Part model, mm, in its own coordinate system. Face numbers are marked on the shaded views. A direction names the side the tool comes from. Coordinates: 2 decimals unless noted, no trailing zeros. Write each loop counter-clockwise with the first axis right and the second up, starting at its lowest first coordinate (ties: lowest second). Pieces come first, ordered by that corner, then holes. Notation, with made-up numbers: M 88.5,84.25 L 139.5,84.25 A24 ccw 139.5,95.25 Z; hole C 57.25,13 d4. An arc over 180 degrees is marked long. Use a Markdown table: item, result. Add a question column.
Q1. Slice it at B-B on z = -24. Write the cut outline in (x, y).
Q2. Wall check: L1, parallel to Y at x = 26, z = 2.5; L2, parallel to Z at x = -24.5, y = 35.5; L3, parallel to Y at x = -27, z = -42. Give the ranges that are in metal, low to high. Write a range as from..to.
Q3. Slice it at A-A on y = 1. Write the cut outline in (x, z), then the cut area to 3 significant figures.
Q4. Slice it at D-D on y = 26. Write the cut outline in (x, z), then the cut area to 3 significant figures.
Q5. Pin check, flat tips, straight feed: pin 1 Ø10 at (x, z) = (-25, -36) entering from -Y; pin 2 Ø24 at (y, z) = (13, 8) entering from -X; pin 3 Ø5 at (y, z) = (-2, -37.5) entering from +X. Stop position of each tip, or through.
Q6. Tool access for the marked faces 5, 6 and 7: list every direction of +Z, -Z, +X, -X, +Y, -Y with a clear straight run to the whole face (end or side of a thin tool).
Q7. Mould opens along Z. For the marked faces 1, 2, 3 and 4 say: released by +Z, released by -Z, zero draft, split by the parting line, or undercut.
Q8. Slice it at C-C on x = -25. Write the cut outline in (y, z).
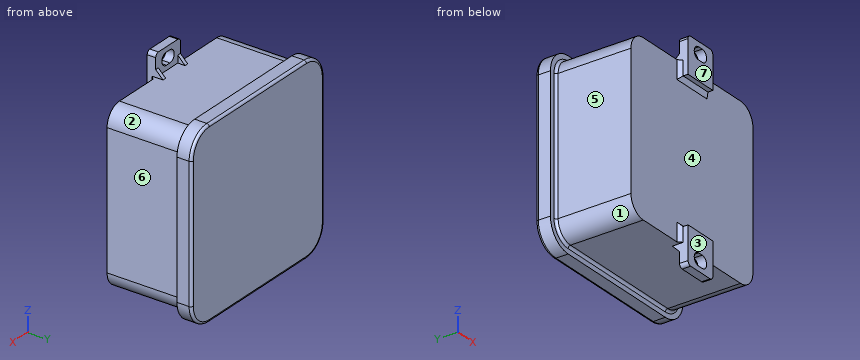
Autodesk Inventor part; units mm, degrees
ref_plane "Work Plane1" through (-1.9723, -3.5, 38.1266) normal (1, 0, 0) x (0, 0, -1)
ref_plane "Work Plane2" through (-29.4723, 30, -5.3734) normal (0, 0, 1) x (1, 0, 0)
ref_plane "YZ Plane" through (0, 0, 0) normal (1, 0, 0) x (0, 1, 0)
sketch "Sketch1" plane through (0, 0, 0) normal (0, 1, 0) x (-1, 0, 0)
  line L0 (36.4723, -39.8734) -> (-32.5277, -39.8734)
  line L1 (-32.5277, -39.8734) -> (-32.5277, 29.1266)
  line L2 (-32.5277, 29.1266) -> (36.4723, 29.1266)
  line L3 (36.4723, 29.1266) -> (36.4723, -39.8734)
  line L4 (36.4723, -39.8734) -> (-32.5277, 29.1266) construction
  line L5 (-32.5277, -39.8734) -> (36.4723, 29.1266) construction
  point P0 (0, 0)
  point P1 (1.9723, -5.3734)
  dimension "d0" = 69
  dimension "d1" = 69
extrude "Extrusion1" add sketch "Sketch1" along normal blind 31
fillet "Fillet1" radius 7 4 edges at (32.5277, 15.5, 29.1266) (-36.4723, 15.5, 29.1266) (-36.4723, 15.5, -39.8734) (32.5277, 15.5, -39.8734)
sketch "Sketch2" plane through (0, 31, 0) normal (0, 1, 0) x (1, 0, 0)
  arc A0 (32.5277, 32.8734) -> (25.5277, 39.8734) centre (25.5277, 32.8734) ccw
  line L0 (25.5277, 39.8734) -> (-29.4723, 39.8734)
  arc A1 (-29.4723, 39.8734) -> (-36.4723, 32.8734) centre (-29.4723, 32.8734) ccw
  line L1 (-36.4723, 32.8734) -> (-36.4723, -22.1266)
  arc A2 (-36.4723, -22.1266) -> (-29.4723, -29.1266) centre (-29.4723, -22.1266) ccw
  line L2 (-29.4723, -29.1266) -> (25.5277, -29.1266)
  arc A3 (25.5277, -29.1266) -> (32.5277, -22.1266) centre (25.5277, -22.1266) ccw
  line L3 (32.5277, -22.1266) -> (32.5277, 32.8734)
  line L4 (-29.4723, 42.8734) -> (25.5277, 42.8734)
  arc A4 (35.5277, 32.8734) -> (25.5277, 42.8734) centre (25.5277, 32.8734) ccw
  line L5 (35.5277, 32.8734) -> (35.5277, -22.1266)
  arc A5 (25.5277, -32.1266) -> (35.5277, -22.1266) centre (25.5277, -22.1266) ccw
  line L6 (25.5277, -32.1266) -> (-29.4723, -32.1266)
  arc A6 (-39.4723, -22.1266) -> (-29.4723, -32.1266) centre (-29.4723, -22.1266) ccw
  line L7 (-39.4723, -22.1266) -> (-39.4723, 32.8734)
  arc A7 (-29.4723, 42.8734) -> (-39.4723, 32.8734) centre (-29.4723, 32.8734) ccw
  point P0 (0, 0)
  dimension "d5" = 3
extrude "Extrusion2" add sketch "Sketch2" along normal blind 6 contours L3 A3 L2 A2 L1 A1 L0 A0 | L4 A4 L5 A5 L6 A6 L7 A7
fillet "Fillet2" radius 1 8 edges at (-1.9723, 31, 29.1266) (-34.422, 31, 27.0763) (-36.4723, 31, -5.3734) (-34.422, 31, -37.8232) (-1.9723, 31, -39.8734) (30.4775, 31, -37.8232) (32.5277, 31, -5.3734) (30.4775, 31, 27.0763)
fillet "Fillet3" radius 1 8 edges at (32.5988, 37, 29.1977) (35.5277, 37, -5.3734) (32.5988, 37, -39.9445) (-1.9723, 37, -42.8734) (-36.5433, 37, -39.9445) (-39.4723, 37, -5.3734) (-36.5433, 37, 29.1977) (-1.9723, 37, 32.1266)
sketch "Sketch3" plane through (0, 0, 0) normal (0, -1, 0) x (1, 0, 0)
  line L0 (32.5277, -32.8734) -> (32.5277, 22.1266)
  line L1 (25.5277, 29.1266) -> (-29.4723, 29.1266)
  line L2 (-36.4723, 22.1266) -> (-36.4723, -32.8734)
  line L3 (-8.9723, 38.1266) -> (5.0277, 38.1266)
  line L4 (5.0277, 38.1266) -> (5.0277, 23.1266)
  line L5 (5.0277, 23.1266) -> (-8.9723, 23.1266)
  line L6 (-8.9723, 23.1266) -> (-8.9723, 38.1266)
  line L7 (-8.9723, 23.1266) -> (-36.4723, 23.1266)
  line L8 (5.0277, 23.1266) -> (32.5277, 23.1266)
  point P0 (0, 0)
  dimension "d10" = 14
  dimension "d12" = 15
  dimension "d13" = 9
extrude "Extrusion3" add sketch "Sketch3" along normal blind 3.5
chamfer "Chamfer1" distance 1.5 angle 45 3 edges at (-8.9723, 0, 26.1266) (-1.9723, 0, 23.1266) (5.0277, 0, 26.1266)
sketch "Sketch4" plane through (0, 0, 0) normal (0, 1, 0) x (1, 0, 0)
  line L0 (5.0277, -29.1266) -> (-8.9723, -29.1266)
  line L1 (-8.9723, -38.1266) -> (5.0277, -38.1266)
  line L2 (-1.9723, -38.1266) -> (-1.9723, -29.1266)
  line L3 (-1.9723, -33.6266) -> (-0.9723, -33.6266)
  line L4 (-1.9723, -33.6266) -> (-2.9723, -33.6266)
  circle A0 centre (-2.9723, -33.6266) radius 2.5
  circle A1 centre (-0.9723, -33.6266) radius 2.5
  line L5 (-2.9723, -31.1266) -> (-0.9723, -31.1266)
  line L6 (-0.9723, -31.1266) -> (-0.9723, -36.1266)
  line L7 (-0.9723, -36.1266) -> (-2.9723, -36.1266)
  line L8 (-2.9723, -36.1266) -> (-2.9723, -31.1266)
  point P0 (0, 0)
  dimension "d21" = 5
  dimension "d22" = 5
  dimension "d19" = 1
  dimension "d20" = 1
extrude "Extrusion4" cut sketch "Sketch4" against normal blind 3.5
sketch "Sketch5" plane through (5.0277, 0, 38.1266) normal (1, 0, 0) x (0, 0, -1)
  line L0 (0, 0) -> (9, 0)
  line L1 (9, 0) -> (9, 30)
  line L2 (9, -1.5) -> (9, 0)
  line L3 (9, 0) -> (9, -1.5)
  line L4 (9, -1.5) -> (9, 0)
  line L5 (9, -1.5) -> (9, 0)
  line L6 (9, 30) -> (9, 0)
  line L7 (6, 0) -> (9, 3)
  line L8 (6, 0) -> (10.2426, 0) construction
  line L9 (6, 0) -> (9, 0)
  line L10 (9, 3) -> (9, 0)
  point P0 (38.1266, 0)
  dimension "d25" = 45
  dimension "d26" = 3
extrude "Extrusion5" add sketch "Sketch5" against normal blind 1.5
ref_plane "Work Plane1" through (-1.9723, -3.5, 38.1266) normal (1, 0, 0) x (0, 0, -1)
mirror "Mirror1" about plane through (-1.9723, -3.5, 38.1266) normal (1, 0, 0) of "Extrusion5"
fillet "Fillet4" radius 1.5 2 edges at (-8.9723, -1.75, 38.1266) (5.0277, -1.75, 38.1266)
ref_plane "Work Plane2" through (-29.4723, 30, -5.3734) normal (0, 0, 1) x (1, 0, 0)
mirror "Mirror2" about plane through (-29.4723, 30, -5.3734) normal (0, 0, 1) of "Extrusion3", "Chamfer1", "Extrusion4", "Extrusion5", "Mirror1", "Fillet4"
ref_plane "Work Plane3" through (-1.9723, -3.5, -48.8734) normal (-1, 0, 0) x (0, 0, 1)
properties part number "power_conduit_box"
Recorded:
| question | item | result |
|---|---|---|
| 1 | outline | M -39.47,31 L -37.47,31 A1 cw -36.47,30 L -36.47,0 L 32.53,0 L 32.53,30 A1 cw 33.53,31 L 35.53,31 L 35.53,36 A1 ccw 34.53,37 L -38.47,37 A1 ccw -39.47,36 Z |
| 2 | L1 | 0..37 |
| 2 | L2 | -42.87..32.13 |
| 2 | L3 | 31..36.99 |
| 3 | outline | M -36.47,-32.87 A7 ccw -29.47,-39.87 L -8.97,-39.87 L -8.97,-41.87 L -7.47,-41.87 L -7.47,-39.87 L 3.53,-39.87 L 3.53,-41.87 L 5.03,-41.87 L 5.03,-39.87 L 25.53,-39.87 A7 ccw 32.53,-32.87 L 32.53,22.13 A7 ccw 25.53,29.13 L 5.03,29.13 L 5.03,31.13 L 3.53,31.13 L 3.53,29.13 L -7.47,29.13 L -7.47,31.13 L -8.97,31.13 L -8.97,29.13 L -29.47,29.13 A7 ccw -36.47,22.13 Z |
| 3 | area | 4,730 mm² |
| 4 | outline | M -36.47,-32.87 A7 ccw -29.47,-39.87 L 25.53,-39.87 A7 ccw 32.53,-32.87 L 32.53,22.13 A7 ccw 25.53,29.13 L -29.47,29.13 A7 ccw -36.47,22.13 Z |
| 4 | area | 4,720 mm² |
| 5 | pin 1 | y = 0 |
| 5 | pin 2 | x = -36.47 |
| 5 | pin 3 | x = 31.79 |
| 6 | face 5 | +Z, -Z, -X, -Y |
| 6 | face 6 | +Z, -Z, +X, -Y |
| 6 | face 7 | +Z, -Z, +X, -X, -Y |
| 7 | face 1 | released by -Z |
| 7 | face 2 | released by +Z |
| 7 | face 3 | zero draft |
| 7 | face 4 | undercut |
| 8 | outline | M 0,-39.87 L 30,-39.87 A1 cw 31,-40.87 L 31,-42.87 L 36,-42.87 A1 ccw 37,-41.87 L 37,31.13 A1 ccw 36,32.13 L 31,32.13 L 31,30.13 A1 cw 30,29.13 L 0,29.13 Z |
